CAD build for the part. Positions are in the model's coordinates, mm. A direction names the side the tool comes from. Give positions to 0.01 mm unless a question says otherwise; leave off trailing zeros. Order: outer loops, then holes, each group sorted by start corner. A loop starts at its lowest first (then second) coordinate and runs counter-clockwise, first axis right, second up. Notation, with made-up numbers: (-21.75, 85) -> (-16.75, 85) arc R21 cw to (-16.75, 122) -> close; hole circle Ø7 at (54.5, 31.5). An arc over 180 degrees is marked (long way). Answer as CSV lines item,"result".
```python
from build123d import *

# Parameters (mm, degrees)
SKETCH2_W           = 20
SKETCH2_H           = 8.6
BOSS_EXTRUDE1_DEPTH = 12
SKETCH3_W           = 28
SKETCH3_H           = 8.6
SKETCH3_R           = 1
BOSS_EXTRUDE2_DEPTH = 1
SKETCH4_W           = 20
SKETCH4_H           = 8.6
BOSS_EXTRUDE3_DEPTH = 2.7
SKETCH5_W           = 18
SKETCH5_H           = 8.6
BOSS_EXTRUDE4_DEPTH = 1.6
BOSS_EXTRUDE5_DEPTH = 3
SKETCH7_R           = 2.75
BOSS_EXTRUDE6_DEPTH = 3
SKETCH8_W           = 0.593912785
SKETCH8_H           = 2.2
BOSS_EXTRUDE7_DEPTH = 5


with BuildPart() as part:
    # Sketch2 → Boss-Extrude1 (new body)
    with BuildSketch(Plane.XY):
        Rectangle(SKETCH2_W, SKETCH2_H)
    extrude(amount=BOSS_EXTRUDE1_DEPTH)

    # Sketch3 → Boss-Extrude2 (add)
    with BuildSketch(Plane.XY.offset(12)):
        Rectangle(SKETCH3_W, SKETCH3_H)
        with Locations((12, 0)):
            Circle(SKETCH3_R, mode=Mode.SUBTRACT)
        with Locations((-12, 0)):
            Circle(SKETCH3_R, mode=Mode.SUBTRACT)
    extrude(amount=BOSS_EXTRUDE2_DEPTH)

    # Sketch4 → Boss-Extrude3 (add)
    with BuildSketch(Plane.XY.offset(13)):
        Rectangle(SKETCH4_W, SKETCH4_H)
    extrude(amount=BOSS_EXTRUDE3_DEPTH)

    # Sketch5 → Boss-Extrude4 (add)
    with BuildSketch(Plane.XY.offset(15.7)):
        with Locations((-1, 0)):
            Rectangle(SKETCH5_W, SKETCH5_H)
    extrude(amount=BOSS_EXTRUDE4_DEPTH)

    # Sketch6 → Boss-Extrude5 (add)
    with BuildSketch(Plane.XY.offset(17.3)):
        with BuildLine():
            Line((-8, 4.3), (1, 4.3))
            Line((1, 4.3), (1, -4.3))
            Line((1, -4.3), (-8, -4.3))
            ThreePointArc((-8, -4.3), (-9.414213562, -3.714213562), (-10, -2.3))
            Line((-10, -2.3), (-10, 2.3))
            ThreePointArc((-10, 2.3), (-9.414213562, 3.714213562), (-8, 4.3))
        make_face()
    extrude(amount=BOSS_EXTRUDE5_DEPTH)

    # Sketch7 → Boss-Extrude6 (add)
    with BuildSketch(Plane.XY.offset(20.3)):
        with Locations((-6, 0)):
            Circle(SKETCH7_R)
    extrude(amount=BOSS_EXTRUDE6_DEPTH)

    # Sketch8 → Boss-Extrude7 (add)
    with BuildSketch(Plane.ZY.offset(10)):
        with Locations((0.296956392, -0.387828177)):
            Rectangle(SKETCH8_W, SKETCH8_H)
    extrude(amount=BOSS_EXTRUDE7_DEPTH)


solid = part.part
```
1) Which spindle directions (+Z, -Z, +X, -X, +Y, -Y) get a long thin tool onto all of the face, cutting with end or side? Do faces 4 (the flat face through (-9.6, -3.8, 17.3)), 5 (the flat face through (-12, 0, 0.594)), 6 (the flat face through (8, 0, 16)), 7 (the flat face through (-14, -0.1, 12.5)). Say none if no direction does.
Data:
face 4,"+Z, -X, -Y"
face 5,"-X, +Y, -Y"
face 6,"+Z, +X, +Y, -Y"
face 7,"+Z, -X, +Y, -Y"
2) Band-saw the part on B-B, the plane y = 0. Give the number of separate pieces and of enclosed holes in the cut face, then the cut area to 3 significant figures.
Data:
separate pieces,"3"
enclosed holes,"0"
area,"399 mm2"
3) Band-saw the part on C-C, the plane x = 12. Write the cut outline in (y, z), then the cut area to 3 significant figures.
Data:
outline,"(-4.3, 12) -> (-1, 12) -> (-1, 13) -> (-4.3, 13) -> close; (1, 12) -> (4.3, 12) -> (4.3, 13) -> (1, 13) -> close"
area,"6.60 mm2"
4) Band-saw the part on D-D, the plane y = 3.5. Write the cut outline in (x, z), then the cut area to 3 significant figures.
Data:
outline,"(-14, 12) -> (-10, 12) -> (-10, 0) -> (10, 0) -> (10, 12) -> (14, 12) -> (14, 13) -> (10, 13) -> (10, 15.7) -> (8, 15.7) -> (8, 17.3) -> (1, 17.3) -> (1, 20.3) -> (-9.6, 20.3) -> (-9.6, 17.3) -> (-10, 17.3) -> (-10, 13) -> (-14, 13) -> close"
area,"383 mm2"
5) Pull direction Y, two halves, no side cores. Call faces 1 (the flat face through (0, -4.3, 10)), 2 (the cylindrical face through (-13, 0, 12.5)), 3 (the flat face through (1, 0, 19)): pulls with the +Y half, pulls with the -Y half, needs draft (parallel to the pull), parting line crosses it, or undercut.
Data:
face 1,"pulls with the -Y half"
face 2,"undercut"
face 3,"needs draft"
6) Band-saw the part on A-A, the plane x = -12. Write the cut outline in (y, z), then the cut area to 3 significant figures.
Data:
outline,"(-4.3, 12) -> (-1, 12) -> (-1, 13) -> (-4.3, 13) -> close; (-1.49, 0) -> (0.71, 0) -> (0.71, 0.59) -> (-1.49, 0.59) -> close; (1, 12) -> (4.3, 12) -> (4.3, 13) -> (1, 13) -> close"
area,"7.91 mm2"
7) Wall check: line 1 along Y through (x, z) = (12, 12.2); line 2 along X through (y, z) = (-2.25, 17.25); line 3 along Z through (x, y) = (0.25, 2). Give the ranges that are in metal, low to high. Write a range as [from, to].
Data:
line 1,"y = [-4.3, -1], [1, 4.3]"
line 2,"x = [-10, 8]"
line 3,"z = [0, 20.3]"
8) Pin check, flat tips, straight feed: P1, Ø0.5, axis at y = -1, z = 16.5, coming from the +X side; P2, Ø2.5, axis at y = -2, z = 19, coming from the +X side; P3, Ø3, axis at x = 12.5, y = 0.5, coming from the -Z side. Stop position of each tip, or through.
Data:
P1,"stops at x = 8"
P2,"stops at x = 1"
P3,"stops at z = 12"
